Read the model definition and answer for the solid it produces. Units are mm, in the model's axes. Face numbers are marked on the shaded views. A direction names the side the tool comes from. Coordinates: 2 decimals unless noted, no trailing zeros. Order: outer loops, then holes, each group sorted by start corner. A loop starts at its lowest first (then second) coordinate and runs counter-clockwise, first axis right, second up.
```python
from build123d import *

# Parameters (mm, degrees)
F1_R      = 35.5
F2_DEPTH  = 8.5
F0_R      = 30.25
F3_DEPTH  = 8.5
F5_W      = 68
F5_H      = 28
F5_H_2    = 30.5
F6_DEPTH  = 60
F7_R      = 35.25
F8_DEPTH  = 2
F9_DEPTH  = 100
F10_R     = 19
F11_DEPTH = 12
F12_R     = 26.1
F13_DEPTH = 9.5
F15_DEPTH = 6.5
F17_DEPTH = 25
F18_R     = 12.84
F19_DEPTH = 10.7
F20_R     = 10.8
F21_DEPTH = 25
F22_R     = 12.84
F23_DEPTH = 7
F24_R     = 0.8
F25_DEPTH = 3
F26_R     = 2.55
F27_DEPTH = 5
F28_R     = 10.8
F29_DEPTH = 25
F30_R     = 12.84
F31_DEPTH = 10.7
F32_R     = 1.13
F33_DEPTH = 6
F34_R     = 1.13
F35_DEPTH = 6


with BuildPart() as f2:
    # F1 (on Top) → F2 (new body)
    with BuildSketch(Plane.XY):
        Circle(F1_R)
    extrude(amount=F2_DEPTH)

    # F0 (on Top) → F3 (cut)
    with BuildSketch(Plane.XY):
        Circle(F0_R)
    extrude(amount=F3_DEPTH, mode=Mode.SUBTRACT)

    # F5 (on face) → F6 (join)
    with BuildSketch(Plane.XY.offset(8.5)):
        with Locations((0, 14)):
            Rectangle(F5_W, F5_H)
        with Locations((0, -15.25)):
            Rectangle(F5_W, F5_H_2)
    extrude(amount=F6_DEPTH)

    # F7 (on face) → F8 (join)
    with BuildSketch(Plane(origin=(0, 0, 8.5), x_dir=(1, 0, 0), z_dir=(0, 0, -1))):
        Circle(F7_R)
    extrude(amount=F8_DEPTH)

    # F4 (on face) → F9 (cut, symmetric)
    with BuildSketch(Plane.XY.offset(8.5)):
        with BuildLine():
            Line((-19.3, -20), (19.3, -20))
            ThreePointArc((19.3, -20), (21.4213203436, -19.1213203436), (22.3, -17))
            Line((22.3, -17), (22.3, 17))
            ThreePointArc((22.3, 17), (21.4213203436, 19.1213203436), (19.3, 20))
            Line((19.3, 20), (-19.3, 20))
            ThreePointArc((-19.3, 20), (-21.4213203436, 19.1213203436), (-22.3, 17))
            Line((-22.3, 17), (-22.3, -17))
            ThreePointArc((-22.3, -17), (-21.4213203436, -19.1213203436), (-19.3, -20))
        make_face()
    extrude(amount=F9_DEPTH, both=True, mode=Mode.SUBTRACT)

    # F10 (on face) → F11 (cut)
    with BuildSketch(Plane.XZ.offset(30.5)):
        with Locations((0, 38.5)):
            Circle(F10_R)
    extrude(amount=-F11_DEPTH, mode=Mode.SUBTRACT)

    # F12 (on face) → F13 (cut)
    with BuildSketch(Plane.XZ.offset(30.5)):
        with Locations((0, 38.5)):
            Circle(F12_R)
    extrude(amount=-F13_DEPTH, mode=Mode.SUBTRACT)

    # F14 (on face) → F15 (cut)
    with BuildSketch(Plane.XZ.offset(30.5)):
        with BuildLine():
            Line((-24.625, 10.875), (24.625, 10.875))
            ThreePointArc((24.625, 10.875), (26.7463203436, 11.7536796564), (27.625, 13.875))
            Line((27.625, 13.875), (27.625, 63.125))
            ThreePointArc((27.625, 63.125), (26.7463203436, 65.2463203436), (24.625, 66.125))
            Line((24.625, 66.125), (-24.625, 66.125))
            ThreePointArc((-24.625, 66.125), (-26.7463203436, 65.2463203436), (-27.625, 63.125))
            Line((-27.625, 63.125), (-27.625, 13.875))
            ThreePointArc((-27.625, 13.875), (-26.7463203436, 11.7536796564), (-24.625, 10.875))
        make_face()
    extrude(amount=-F15_DEPTH, mode=Mode.SUBTRACT)

    # F16 (on face) → F17 (cut)
    with BuildSketch(Plane(origin=(-34, 0, 0), x_dir=(0, -1, 0), z_dir=(-1, 0, 0))):
        with BuildLine():
            ThreePointArc((0, 27.7), (7.6367532368, 30.8632467632), (10.8, 38.5))
            ThreePointArc((10.8, 38.5), (-7.6367532368, 46.1367532368), (0, 27.7))
        make_face()
    extrude(amount=-F17_DEPTH, mode=Mode.SUBTRACT)

    # F18 (on face) → F19 (cut)
    with BuildSketch(Plane(origin=(-34, 0, 0), x_dir=(0, -1, 0), z_dir=(-1, 0, 0))):
        with Locations((0, 38.5)):
            Circle(F18_R)
    extrude(amount=-F19_DEPTH, mode=Mode.SUBTRACT)

    # F20 (on face) → F21 (cut)
    with BuildSketch(Plane(origin=(0, 28, 0), x_dir=(-1, 0, 0), z_dir=(0, 1, 0))):
        with Locations((0, 38.5)):
            Circle(F20_R)
    extrude(amount=-F21_DEPTH, mode=Mode.SUBTRACT)

    # F22 (on face) → F23 (cut)
    with BuildSketch(Plane(origin=(0, 28, 0), x_dir=(-1, 0, 0), z_dir=(0, 1, 0))):
        with Locations((0, 38.5)):
            Circle(F22_R)
    extrude(amount=-F23_DEPTH, mode=Mode.SUBTRACT)

    # F24 (on face) → F25 (cut)
    with BuildSketch(Plane.XZ.offset(24)):
        with Locations((-22, 60.5)):
            Circle(F24_R)
        with Locations((22, 60.5)):
            Circle(F24_R)
        with Locations((22, 16.5)):
            Circle(F24_R)
        with Locations((-22, 16.5)):
            Circle(F24_R)
    extrude(amount=-F25_DEPTH, mode=Mode.SUBTRACT)

    # F26 (on face) → F27 (cut)
    with BuildSketch(Plane(origin=(0, 28, 0), x_dir=(-1, 0, 0), z_dir=(0, 1, 0))):
        with Locations((-25.4, 55)):
            Circle(F26_R)
        with Locations((25.4, 55)):
            Circle(F26_R)
        with Locations((25.4, 22)):
            Circle(F26_R)
        with Locations((-25.4, 22)):
            Circle(F26_R)
    extrude(amount=-F27_DEPTH, mode=Mode.SUBTRACT)

    # F28 (on face) → F29 (cut)
    with BuildSketch(Plane.YZ.offset(34)):
        with Locations((0, 38.5)):
            Circle(F28_R)
    extrude(amount=-F29_DEPTH, mode=Mode.SUBTRACT)

    # F30 (on face) → F31 (cut)
    with BuildSketch(Plane.YZ.offset(34)):
        with Locations((0, 38.5)):
            Circle(F30_R)
    extrude(amount=-F31_DEPTH, mode=Mode.SUBTRACT)

    # F32 (on face) → F33 (cut)
    with BuildSketch(Plane.YZ.offset(34)):
        with Locations((-15, 53.5)):
            Circle(F32_R)
        with Locations((15, 53.5)):
            Circle(F32_R)
        with Locations((15, 23.5)):
            Circle(F32_R)
        with Locations((-15, 23.5)):
            Circle(F32_R)
    extrude(amount=-F33_DEPTH, mode=Mode.SUBTRACT)

    # F34 (on face) → F35 (cut)
    with BuildSketch(Plane(origin=(-34, 0, 0), x_dir=(0, -1, 0), z_dir=(-1, 0, 0))):
        with Locations((-15, 23.5)):
            Circle(F34_R)
        with Locations((15, 23.5)):
            Circle(F34_R)
        with Locations((15, 53.5)):
            Circle(F34_R)
        with Locations((-15, 53.5)):
            Circle(F34_R)
    extrude(amount=-F35_DEPTH, mode=Mode.SUBTRACT)


solid = f2.part
```
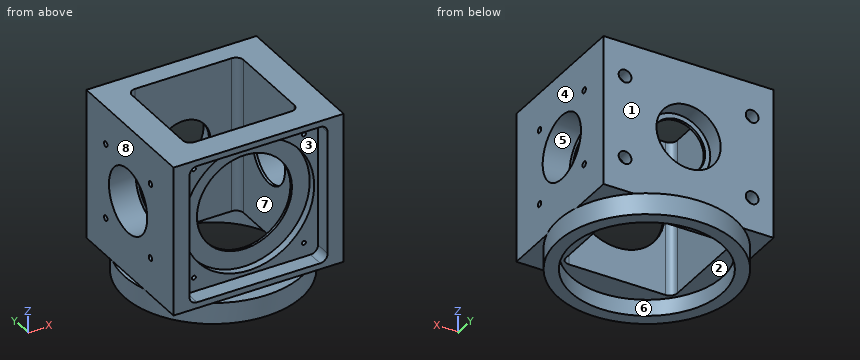
1) Determine the mould class of the marked faces 1, 2, 3 and 4 for opening direction Y: pulls with the +Y half, pulls with the -Y half, needs draft (parallel to the pull), parting line crosses it, or undercut.
A:
face 1: pulls with the +Y half
face 2: undercut
face 3: pulls with the -Y half
face 4: needs draft
2) Which of the six approach directions +Z, -Z, +X, -X, +Y, -Y give full straight-line access (tool end or side, diameter ignored) to the marked faces 5, 6, 7 and 8?
A:
face 5: +X
face 6: -Z
face 7: +Z, -Z
face 8: +Z, -X, +Y, -Y
3) Straight lines are drawn through the part: line 1 (Z direction, x = 25.4, y = 26.9); line 2 (Z direction, x = 25.4, y = 24.5); line 3 (Z direction, x = 31, y = 0). For each, find the intervals that lie inside material, in ascending order.
A:
line 1: z = 8.5 to 19.45, 24.55 to 52.45, 57.55 to 68.5
line 2: z = 0 to 19.45, 24.55 to 52.45, 57.55 to 68.5
line 3: z = 0 to 25.66, 51.34 to 68.5
4) A cutting plane is placed at B-B, the plane y = -3. State how many separate pieces and enclosed holes the cut face has, and give its area (3 significant figures).
A:
separate pieces: 4
enclosed holes: 0
area: 949 mm2
5) A cutting plane is placed at A-A, the plane x = 16.5. Determine the outline of the cut face in (y, z) (3 decimals).
A:
outline: (-31.432, 0) - (-25.354, 0) - (-25.354, 6.5) - (-20, 6.5) - (-20, 29.079) - (-21, 29.079) - (-21, 18.277) - (-24, 18.277) - (-24, 10.875) - (-30.5, 10.875) - (-30.5, 8.5) - (-31.432, 8.5) - close; (-30.5, 66.125) - (-24, 66.125) - (-24, 58.723) - (-21, 58.723) - (-21, 47.921) - (-20, 47.921) - (-20, 68.5) - (-30.5, 68.5) - close; (20, 6.5) - (25.354, 6.5) - (25.354, 0) - (31.432, 0) - (31.432, 8.5) - (28, 8.5) - (28, 68.5) - (20, 68.5) - close
6) Flat-ended cylindrical pins translate along their axes: pin 1 Ø10 at (x, z) = (25, 18) entering from +Y; pin 2 Ø25 at (y, z) = (0, 38.5) entering from +X; pin 3 Ø1.3 at (x, z) = (22.5, 16.5) entering from -Y; pin 4 Ø8.5 at (x, y) = (7, 32) entering from +Z. Find the tip coordinate at first contact, or state that the pin passes through.
A:
pin 1: stops at y = 28
pin 2: stops at x = 23.3
pin 3: stops at y = -24
pin 4: stops at z = 68.5
